Can you work these out from the model? Positions are in its coordinate system, mm. Round coordinates to 2 decimals unless told otherwise and drop trailing zeros. Write each loop counter-clockwise with the first axis right and the second up, starting at its lowest first coordinate (ties: lowest second). Pieces come first, ordered by that corner, then holes. Notation, with made-up numbers: (-27.5, 52) -> (-3.5, 52) arc R22 ccw to (-3.5, 65) -> close; hole circle Ø4 at (-13.5, -17). An arc over 180 degrees is marked (long way). Write item = value, one per line. Start each with the question number.
1) If I drill on line 1 (Z direction, x = 0.6, y = 26); line 2 (Z direction, x = 1.85, y = 31.5); line 3 (Y direction, x = 1.45, z = -395.5), over which ranges is the centre line in solid material (lowest first)?
2) Imagine slicing it at C-C, the plane x = 1.2. Please give me the cut outline in (y, z).
3) Imagine slicing it at A-A, the plane z = -241. Please give me the cut outline in (x, y).
4) Imagine slicing it at B-B, the plane y = 25. Please give me the cut outline in (x, z).
Autodesk Inventor part; units mm, degrees
ref_plane "YZ Plane" through (0, 0, 0) normal (1, 0, 0) x (0, 1, 0)
ref_plane "XZ Plane" through (0, 0, 0) normal (0, 1, 0) x (-1, 0, 0)
ref_plane "XY Plane" through (0, 0, 0) normal (0, 0, 1) x (1, 0, 0)
sketch "Sketch1" plane through (0, 0, 0) normal (1, 0, 0) x (0, 1, 0)
  line L0 (0, 0) -> (50, 0)
  line L1 (50, 0) -> (50, -500)
  line L2 (50, -500) -> (0, -500)
  line L3 (0, -500) -> (0, 0)
  dimension "d0" = 50
  dimension "d1" = 500
extrude "Plate1" add sketch "Sketch1" along normal blind 3
sketch "Sketch2" plane through (3, 0, 0) normal (1, 0, 0) x (0, 0, -1)
  line L0 (0, 50) -> (0, 0)
  line L1 (0, 25) -> (100, 25)
  line L2 (500, 0) -> (500, 50)
  line L3 (500, 25) -> (400, 25)
  line L4 (100, 25) -> (400, 25)
  line L5 (80.0463, 25) -> (119.9537, 25) construction
  line L6 (80.0463, 17.6266) -> (119.9537, 17.6266)
  line L7 (119.9537, 32.3734) -> (80.0463, 32.3734)
  arc A0 (80.0463, 32.3734) -> (80.0463, 17.6266) centre (80.0463, 25) ccw
  arc A1 (119.9537, 17.6266) -> (119.9537, 32.3734) centre (119.9537, 25) ccw
  line L8 (270.0297, 25) -> (229.9703, 25) construction
  line L9 (270.0297, 17.6266) -> (229.9703, 17.6266)
  line L10 (229.9703, 32.3734) -> (270.0297, 32.3734)
  arc A2 (270.0297, 17.6266) -> (270.0297, 32.3734) centre (270.0297, 25) ccw
  arc A3 (229.9703, 32.3734) -> (229.9703, 17.6266) centre (229.9703, 25) ccw
  line L11 (420.3445, 25) -> (379.6555, 25) construction
  line L12 (420.3445, 17.6266) -> (379.6555, 17.6266)
  line L13 (379.6555, 32.3734) -> (420.3445, 32.3734)
  arc A4 (420.3445, 17.6266) -> (420.3445, 32.3734) centre (420.3445, 25) ccw
  arc A5 (379.6555, 32.3734) -> (379.6555, 17.6266) centre (379.6555, 25) ccw
  point P0 (250, 25)
  dimension "d3" = 100
  dimension "d4" = 100
extrude "Cut1" cut sketch "Sketch2" against normal blind 3
equation "\"d5\" = Thickness"
equation "\"d2\" = Thickness"
equation "\"BendRadius\" = Thickness"
equation "\"BendReliefWidth\" = Thickness"
equation "\"BendReliefDepth\" = 0.5 * Thickness"
equation "\"CornerReliefSize\" = 4 * Thickness"
equation "\"MinimumRemnant\" = 2 * Thickness"
equation "\"TransitionRadius\" = BendRadius"
equation "\"JacobiRadiusSize\" = BendRadius"
equation "\"GapSize\" = Thickness"
properties part number "FLoor Frame, Small" material "Aluminum 6061"
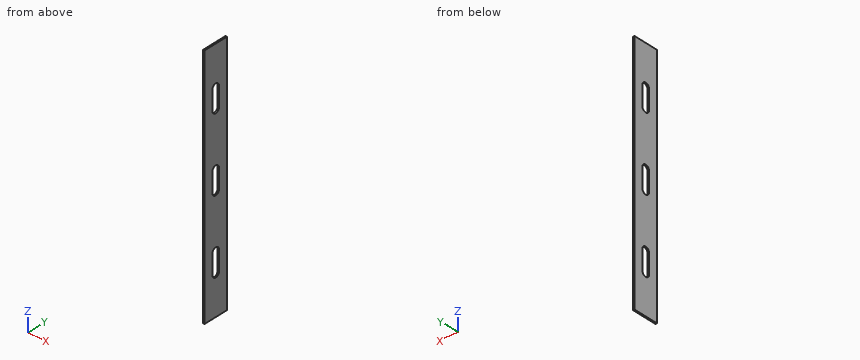
Reported:
q1.line_1 = -500 to -427.65, -372.35 to -277.33, -222.67 to -127.26, -72.74 to 0
q1.line_2 = -500 to -423.83, -376.17 to -273.51, -226.49 to -123.43, -76.57 to 0
q1.line_3 = 0 to 17.63, 32.37 to 50
q2.outline = (0, -500) -> (50, -500) -> (50, 0) -> (0, 0) -> close; hole (17.63, -420.34) arc R7.37 ccw to (32.37, -420.34) -> (32.37, -379.66) arc R7.37 ccw to (17.63, -379.66) -> close; hole (17.63, -270.03) arc R7.37 ccw to (32.37, -270.03) -> (32.37, -229.97) arc R7.37 ccw to (17.63, -229.97) -> close; hole (17.63, -119.95) arc R7.37 ccw to (32.37, -119.95) -> (32.37, -80.05) arc R7.37 ccw to (17.63, -80.05) -> close
q3.outline = (0, 0) -> (3, 0) -> (3, 17.63) -> (0, 17.63) -> close; (0, 32.37) -> (3, 32.37) -> (3, 50) -> (0, 50) -> close
q4.outline = (0, -500) -> (3, -500) -> (3, -427.72) -> (0, -427.72) -> close; (0, -372.28) -> (3, -372.28) -> (3, -277.4) -> (0, -277.4) -> close; (0, -222.6) -> (3, -222.6) -> (3, -127.33) -> (0, -127.33) -> close; (0, -72.67) -> (3, -72.67) -> (3, 0) -> (0, 0) -> close
